Part model, mm, in its own coordinate system. Face numbers are marked on the shaded views. A direction names the side the tool comes from. Round coordinates to 2 decimals unless told otherwise and drop trailing zeros. Order: outer loops, then holes, each group sorted by start corner. A loop starts at its lowest first (then second) coordinate and runs counter-clockwise, first axis right, second up. Notation, with made-up numbers: M -32,50.25 L -27,50.25 A32 cw -27,87.25 Z; hole C 57,23.25 d2. An arc over 180 degrees is marked long. Write each question's results on one line, items separated by ' | '. Start each with the question number.
1. Band-saw the part on C-C, the plane y = 22.5. List the corners of the cut face in (x, z), then the cut area to 3 significant figures.
2. Band-saw the part on D-D, the plane x = 0. List the corners of the cut face in (y, z).
3. Two-plate mould, pull along X, no slides. Class the marked faces 1, 2 and 3: +X half, -X half, draft (parallel to the pull), parting line (faces both ways), or undercut.
4. Which spindle directions (+Z, -Z, +X, -X, +Y, -Y) get a long thin tool onto all of the face, cutting with end or side? Do the marked faces 4, 5, 6 and 7. Say none if no direction does.
5. Drop flat-ended pins along their axis: pin 1 Ø1 at (y, z) = (13, 28) entering from +X; pin 2 Ø5 at (y, z) = (8.5, 3) entering from -X; pin 3 Ø10 at (x, y) = (7, 22) entering from +Z. Give the stop position or say it passes through.
6. Band-saw the part on B-B, the plane z = 9. List the corners of the cut face in (x, y).
7. Band-saw the part on A-A, the plane x = 23. List the corners of the cut face in (y, z), then the cut area to 3 significant figures.
8. Probe L1, parallel to Z at x = -23, y = 21; L2, parallel to X at y = 23, z = -13; L3, parallel to Z at x = 3.5, y = 6.5. List the from-to ranges inside material, lowest first. Write a range as [from, to].
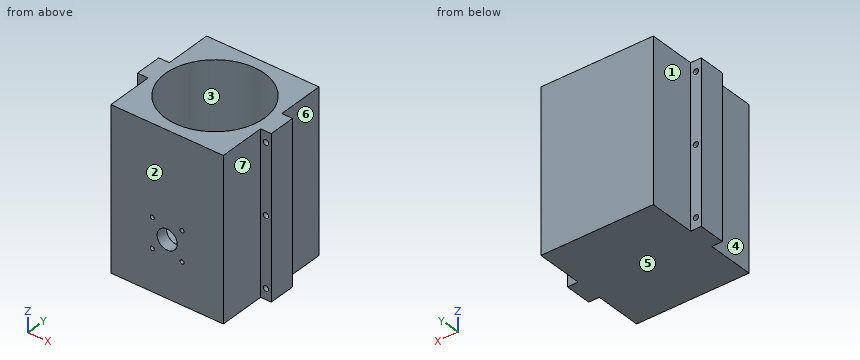
Autodesk Inventor part; units mm, degrees
ref_plane "YZ Plane" through (0, 0, 0) normal (1, 0, 0) x (0, 1, 0)
ref_plane "XZ Plane" through (0, 0, 0) normal (0, 1, 0) x (-1, 0, 0)
ref_plane "XY Plane" through (0, 0, 0) normal (0, 0, 1) x (1, 0, 0)
sketch "Sketch1" plane through (0, 0, 0) normal (0, 1, 0) x (-1, 0, 0)
  circle A0 centre (0, 0) radius 11 construction
  circle A1 centre (0, 0) radius 3.75
  circle A2 centre (0, 0) radius 7.875 construction
  line L0 (16.292, 0) -> (-19, 0) construction
  line L1 (0, 21) -> (0, -27.3544) construction
  line L2 (0, -21) -> (21, -21)
  line L3 (0, -21) -> (-21, -21)
  line L4 (0, 0) -> (21, -21) construction
  circle A3 centre (5.5685, -5.5685) radius 0.75
  circle A4 centre (-5.5685, -5.5685) radius 0.75
  circle A5 centre (5.5685, 5.5685) radius 0.75
  circle A6 centre (-5.5685, 5.5685) radius 0.75
  line L5 (-25, -21) -> (-21, -21)
  line L6 (25, -21) -> (21, -21)
  circle A7 centre (23, -17) radius 1
  circle A8 centre (-23, -17) radius 1
  line L7 (-25, 39) -> (25, 39)
  line L8 (25, -21) -> (25, 39)
  line L9 (21, -21) -> (21, 39)
  line L10 (-21, -21) -> (-21, 39)
  line L11 (-25, -21) -> (-25, 39)
  line L12 (25, 9) -> (-25, 9) construction
  circle A9 centre (23, 35) radius 1
  circle A10 centre (-23, 35) radius 1
  circle A11 centre (23, 9) radius 1
  circle A12 centre (-23, 9) radius 1
  circle A13 centre (5.5685, 5.5685) radius 1.5
  circle A14 centre (5.5685, -5.5685) radius 1.5
  circle A15 centre (-5.5685, 5.5685) radius 1.5
  circle A16 centre (-5.5685, -5.5685) radius 1.5
  dimension "d8" = 15.75
  dimension "d2" = 7.5
  dimension "d4" = 22
  dimension "d17" = 21
  dimension "d26" = 1.5
  dimension "d38" = 60
  dimension "d39" = 21
  dimension "d40" = 2
  dimension "d41" = 2
  dimension "d53" = 3
extrude "Extrusion9" add sketch "Sketch1" along normal blind 45 contours A1 | L3 L10 L7 L9 L2 | A3 | A4 | A5 | A6 | A13 | A14 | A15 | A16
extrude "Extrusion10" add sketch "Sketch1" along normal blind 27.5 contours L9 L7 L8 L6 | L5 L11 L7 L10
extrude "Extrusion11" cut sketch "Sketch1" along normal blind 17.5 contours L9 L7 L8 L6 | L5 L11 L7 L10
extrude "Extrusion13" cut sketch "Sketch1" along normal blind 6 contours A1 | A3 | A4 | A5 | A6 | A13 | A14 | A15 | A16
extrude "Extrusion15" add sketch "Sketch1" along normal blind 3.5 contours A13 | A14 | A15 | A16
sketch "Sketch5" plane through (-21, 45, 39) normal (0, 0, 1) x (1, 0, 0)
  line L0 (0, -45) -> (42, -45) construction
  line L1 (0, -17.5) -> (0, 0) construction
  line L2 (42, -45) -> (0, -45) construction
  line L3 (0, -45) -> (0, 0) construction
  line L4 (0, 0) -> (42, 0) construction
  line L5 (42, 0) -> (42, -45) construction
  line L6 (42, 0) -> (0, -45) construction
  line L7 (0, 0) -> (42, 0) construction
  line L8 (0, 0) -> (42, -45) construction
  circle A0 centre (21, -22.5) radius 18.5
  point P0 (21, -45)
  dimension "d58" = 37
extrude "Extrusion16" cut sketch "Sketch5" against normal blind 55
equation "\"d41\" = d40"
properties part number "engine_connector_sleeve"
Solution:
1) outline: M -25,-21 L 25,-21 L 25,39 L 18.5,39 L 18.5,-16 L -18.5,-16 L -18.5,39 L -25,39 Z; hole C -23,-17 d2; hole C -23,9 d2; hole C -23,35 d2; hole C 23,-17 d2; hole C 23,9 d2; hole C 23,35 d2 | area: 946 mm^2
2) outline: M 0,-21 L 45,-21 L 45,39 L 41,39 L 41,-16 L 4,-16 L 4,-3.75 L 0,-3.75 Z; M 0,3.75 L 4,3.75 L 4,39 L 0,39 Z
3) face 1: -X half | face 2: draft | face 3: undercut
4) face 4: +Z, -Z, -X, -Y | face 5: -Z, +X, -X, +Y, -Y | face 6: +Z, -Z, +X, +Y | face 7: +Z, -Z, +X, -Y
5) pin 1: x = 21 | pin 2: x = -21 | pin 3: z = -16
6) outline: M -25,17.5 L -24,17.5 L -24,27.5 L -25,27.5 Z; M -22,17.5 L -21,17.5 L -21,0 L 21,0 L 21,17.5 L 22,17.5 L 22,27.5 L 21,27.5 L 21,45 L -21,45 L -21,27.5 L -22,27.5 Z; M 24,17.5 L 25,17.5 L 25,27.5 L 24,27.5 Z; hole C 0,22.5 d37
7) outline: M 17.5,-21 L 27.5,-21 L 27.5,-18 L 17.5,-18 Z; M 17.5,-16 L 27.5,-16 L 27.5,8 L 17.5,8 Z; M 17.5,10 L 27.5,10 L 27.5,34 L 17.5,34 Z; M 17.5,36 L 27.5,36 L 27.5,39 L 17.5,39 Z | area: 540 mm^2
8) L1: [-21, -18], [-16, 8], [10, 34], [36, 39] | L2: [-25, -18.49], [18.49, 25] | L3: [-21, -16]
